Autodesk Inventor part; units mm, degrees
ref_plane "YZ Plane" through (0, 0, 0) normal (1, 0, 0) x (0, 1, 0)
ref_plane "XZ Plane" through (0, 0, 0) normal (0, 1, 0) x (-1, 0, 0)
ref_plane "XY Plane" through (0, 0, 0) normal (0, 0, 1) x (1, 0, 0)
sketch "Sketch1" plane through (0, 0, 0) normal (0, 0, 1) x (1, 0, 0)
  line L0 (0, 0) -> (20, 0)
  line L1 (20, 0) -> (20, 41)
  line L2 (20, 41) -> (0, 41)
  line L3 (0, 41) -> (0, 0)
  dimension "d0" = 20
  dimension "d1" = 41
extrude "Extrusion1" add sketch "Sketch1" along normal blind 27
sketch "Sketch2" plane through (0, 0, 27) normal (0, 0, 1) x (1, 0, 0)
  line L0 (0, 41) -> (0, 0) construction
  line L1 (20, 0) -> (20, 41) construction
  line L2 (0, 0) -> (20, 41) construction
  line L3 (20, 41) -> (0, 41) construction
  line L4 (0, 41) -> (20, 0) construction
  line L5 (0, -7) -> (20, -7)
  line L6 (20, -7) -> (20, 48)
  line L7 (20, 48) -> (0, 48)
  line L8 (0, 48) -> (0, -7)
  line L9 (0, -7) -> (20, 48) construction
  line L10 (20, -7) -> (0, 48) construction
  line L11 (0, 41) -> (0, 45) construction
  line L12 (0, 45) -> (20, 45) construction
  line L13 (0, 45) -> (4, 45) construction
  circle A0 centre (4, 45) radius 2
  line L14 (20, 45) -> (16, 45) construction
  circle A1 centre (16, 45) radius 2
  line L15 (0, 0) -> (20, 0) construction
  line L16 (0, 0) -> (0, -4) construction
  line L17 (0, -4) -> (4, -4) construction
  line L18 (20, 0) -> (20, -4) construction
  line L19 (20, -4) -> (16, -4) construction
  circle A2 centre (4, -4) radius 2
  circle A3 centre (16, -4) radius 2
  point P0 (10, 20.5)
  dimension "d4" = 20
  dimension "d5" = 55
  dimension "d6" = 4
  dimension "d7" = 4
  dimension "d8" = 4
  dimension "d9" = 4
  dimension "d10" = 4
  dimension "d11" = 4
  dimension "d12" = 4
  dimension "d13" = 4
  dimension "d14" = 4
  dimension "d15" = 4
  dimension "d16" = 4
extrude "Extrusion2" add sketch "Sketch2" along normal blind 3
sketch "Sketch3" plane through (0, 0, 30) normal (0, 0, 1) x (1, 0, 0)
  line L0 (0, 48) -> (0, 41) construction
  line L1 (0, -7) -> (20, -7) construction
  line L2 (0, 48) -> (20, -7) construction
  line L3 (20, 41) -> (20, 48) construction
  line L4 (0, -7) -> (20, 48) construction
  line L5 (0, 0) -> (20, 0)
  line L6 (20, 0) -> (20, 41)
  line L7 (20, 41) -> (0, 41)
  line L8 (0, 41) -> (0, 0)
  line L9 (0, 0) -> (20, 41) construction
  line L10 (20, 0) -> (0, 41) construction
  point P0 (10, 20.5)
  dimension "d19" = 20
  dimension "d20" = 41
extrude "Extrusion3" add sketch "Sketch3" along normal blind 6
sketch "Sketch4" plane through (0, 0, 36) normal (0, 0, 1) x (1, 0, 0)
  line L0 (20, 48) -> (0, 48) construction
  line L1 (10, 48) -> (10, 30) construction
  circle A0 centre (10, 30) radius 4
  point P0 (0, 0)
  dimension "d23" = 18
  dimension "d24" = 8
extrude "Extrusion4" add sketch "Sketch4" along normal blind 8
sketch "Sketch5" plane through (10, 30, 44) normal (0, 0, 1) x (1, 0, 0)
  line L0 (19.5, -0.7059) -> (19.5, 0.7059)
  line L1 (-19.5, 0.7059) -> (-19.5, -0.7059)
  line L2 (-19.5, -4.5) -> (19.5, 4.5) construction
  line L3 (19.5, -4.5) -> (-19.5, 4.5) construction
  line L4 (-0.7059, 19.5) -> (0.7059, 19.5)
  line L5 (0.7059, -19.5) -> (-0.7059, -19.5)
  line L6 (-4.5, 19.5) -> (4.5, -19.5) construction
  line L7 (4.5, 19.5) -> (-4.5, -19.5) construction
  line L8 (4.5, 7.5) -> (4.5, 6.5)
  line L9 (4.5, -6.5) -> (4.5, -7.5)
  line L10 (-4.5, -7.5) -> (-4.5, -6.5)
  line L11 (-4.5, 6.5) -> (-4.5, 7.5)
  line L12 (-7.5, -4.5) -> (-6.5, -4.5)
  line L13 (6.5, -4.5) -> (7.5, -4.5)
  line L14 (7.5, 4.5) -> (6.5, 4.5)
  line L15 (-6.5, 4.5) -> (-7.5, 4.5)
  arc A0 (-6.5, 4.5) -> (-4.5, 6.5) centre (-6.5, 6.5) ccw
  arc A1 (4.5, 6.5) -> (6.5, 4.5) centre (6.5, 6.5) ccw
  arc A2 (6.5, -4.5) -> (4.5, -6.5) centre (6.5, -6.5) ccw
  arc A3 (-4.5, -6.5) -> (-6.5, -4.5) centre (-6.5, -6.5) ccw
  line L16 (4.5, 7.5) -> (2.6755, 17.8473)
  line L17 (-4.5, 7.5) -> (-2.6755, 17.8473)
  line L18 (7.5, -4.5) -> (17.8473, -2.6755)
  line L19 (7.5, 4.5) -> (17.8473, 2.6755)
  line L20 (-7.5, 4.5) -> (-17.8473, 2.6755)
  line L21 (-7.5, -4.5) -> (-17.8473, -2.6755)
  line L22 (-4.5, -7.5) -> (-2.6755, -17.8473)
  line L23 (4.5, -7.5) -> (2.6755, -17.8473)
  arc A4 (-17.8473, 2.6755) -> (-19.5, 0.7059) centre (-17.5, 0.7059) ccw
  arc A5 (-19.5, -0.7059) -> (-17.8473, -2.6755) centre (-17.5, -0.7059) ccw
  arc A6 (-0.7059, 19.5) -> (-2.6755, 17.8473) centre (-0.7059, 17.5) ccw
  arc A7 (2.6755, 17.8473) -> (0.7059, 19.5) centre (0.7059, 17.5) ccw
  arc A8 (19.5, 0.7059) -> (17.8473, 2.6755) centre (17.5, 0.7059) ccw
  arc A9 (17.8473, -2.6755) -> (19.5, -0.7059) centre (17.5, -0.7059) ccw
  arc A10 (-2.6755, -17.8473) -> (-0.7059, -19.5) centre (-0.7059, -17.5) ccw
  arc A11 (0.7059, -19.5) -> (2.6755, -17.8473) centre (0.7059, -17.5) ccw
  point P0 (-10, -30)
  point P1 (0, 0)
  point P2 (0, 0)
  dimension "d27" = 39
  dimension "d28" = 9
  dimension "d29" = 9
  dimension "d30" = 39
  dimension "d31" = 29.5
  dimension "d32" = 49.5
  dimension "d33" = 2
  dimension "d34" = 12
  dimension "d35" = 10
  dimension "d36" = 12
  dimension "d37" = 10
  dimension "d38" = 12
  dimension "d39" = 10
  dimension "d40" = 12
  dimension "d41" = 10
  dimension "d42" = 12
  dimension "d43" = 10
  dimension "d44" = 12
  dimension "d45" = 10
  dimension "d46" = 12
  dimension "d47" = 10
  dimension "d48" = 12
  dimension "d49" = 10
  dimension "d50" = 2
  dimension "d51" = 2
extrude "Extrusion5" add sketch "Sketch5" against normal blind 2
equation "\"d36\" = d34"
equation "\"d37\" = d35"
equation "\"d38\" = d34"
equation "\"d39\" = d35"
equation "\"d40\" = d34"
equation "\"d41\" = d35"
equation "\"d42\" = d34"
equation "\"d43\" = d35"
equation "\"d44\" = d34"
equation "\"d45\" = d35"
equation "\"d46\" = d34"
equation "\"d47\" = d35"
equation "\"d48\" = d34"
equation "\"d49\" = d35"
properties part number "FutabaS3003Rough" material "PC/ABS Plastic"
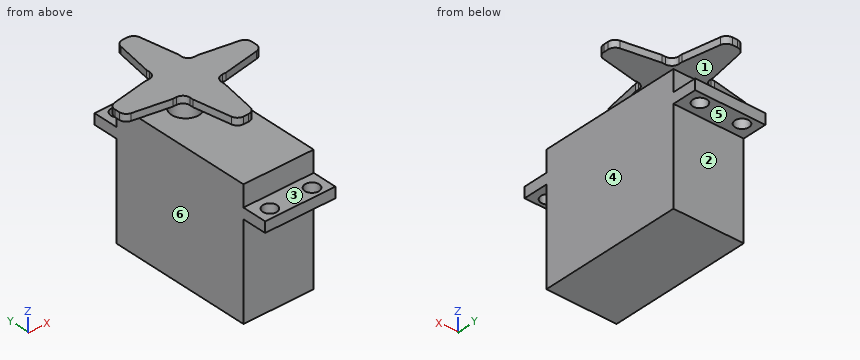
Could you check a few things on this model? Use its own coordinates, in mm. Face numbers are marked on the shaded views. A direction names the side the tool comes from. Give positions to 0.01 mm unless a question says otherwise; leave off trailing zeros. Loops run counter-clockwise (first coordinate to the right, second up) from the corner with the lowest first, then second, coordinate; pieces in that order, holes last. Notation, with made-up numbers: (17.25, 1.25) - (65.25, 1.25) arc R33 cw to (65.25, 34.25) - close; hole circle Ø5 at (17.5, 18). An arc over 180 degrees is marked (long way). Answer in a Markdown table with one row per item. Add a question column.
Q1. We'd pull the mould along X, two halves only. Please class the marked faces 4, 5 and 6: +X half, -X half, draft (parallel to the pull), parting line (faces both ways), or undercut.
Q2. If we section it at C-C (z = 31.5): List the corners of the cut face in (x, y) for me, plus the area to 3 significant figures.
Q3. If we section it at B-B (y = 45): List the corners of the cut face in (x, z) for me.
Q4. Please list where these lines run through material, in increasing order: L1, parallel to Y at x = 16, z = 29.4; L2, parallel to Z at x = 8, y = 37; L3, parallel to X at y = 13.5, z = 14.5. Write a range as from..to.
Q5. If we section it at D-D (y = 30): List the corners of the cut face in (x, z) for me, plus the area to 3 significant figures.
Q6. For pin 1 (2 mm diameter, centred on x = 9, y = 43.5, fed in from -Z); pin 2 (6 mm diameter, centred on x = 10.5, z = 11.5, fed in from -Y); pin 3 (1.1 mm diameter, centred on y = 37, z = 43, fed in from -X), each with a flat end and sliding along its axis, tell me the tip position at first contact or that it passes through.
Q7. If we section it at A-A (y = -4): List the corners of the cut face in (x, z) for me.
Q8. Which directions (+Z, -Z, +X, -X, +Y, -Y) give clear straight access to the entire face, cutting with the end or side of a thin tool? Please do the marked faces 1, 2 and 3.
The answers:
| question | item | result |
|---|---|---|
| 1 | face 4 | +X half |
| 1 | face 5 | draft |
| 1 | face 6 | -X half |
| 2 | outline | (0, 0) - (20, 0) - (20, 41) - (0, 41) - close |
| 2 | area | 820 mm^2 |
| 3 | outline | (0, 27) - (2, 27) - (2, 30) - (0, 30) - close; (6, 27) - (14, 27) - (14, 30) - (6, 30) - close; (6.82, 42) - (13.18, 42) - (13.18, 44) - (6.82, 44) - close; (18, 27) - (20, 27) - (20, 30) - (18, 30) - close |
| 4 | L1 | y = -7..-6, -2..43, 47..48 |
| 4 | L2 | z = 0..36, 42..44 |
| 4 | L3 | x = 0..20 |
| 5 | outline | (-9.5, 42) - (6, 42) - (6, 36) - (0, 36) - (0, 0) - (20, 0) - (20, 36) - (14, 36) - (14, 42) - (29.5, 42) - (29.5, 44) - (-9.5, 44) - close |
| 5 | area | 846 mm^2 |
| 6 | pin 1 | stops at z = 27 |
| 6 | pin 2 | stops at y = 0 |
| 6 | pin 3 | stops at x = 5.5 |
| 7 | outline | (0, 27) - (2, 27) - (2, 30) - (0, 30) - close; (6, 27) - (14, 27) - (14, 30) - (6, 30) - close; (18, 27) - (20, 27) - (20, 30) - (18, 30) - close |
| 8 | face 1 | none |
| 8 | face 2 | -Z, +X, -X, +Y |
| 8 | face 3 | +Z, +X, -X, -Y |
